```python
from build123d import *

# Parameters (mm, degrees)
F1_DEPTH = 50
F3_D     = 4.25


# Not quite as in the source:
# - a feature names something its author has since deleted; it is built from what else it names


with BuildPart() as f1:
    # F0 (on Top) → F1 (new body)
    with BuildSketch(Plane.XY):
        Polygon((-30.2708722231, 4.5814236456), (-30.2708722231, 0), (-30.2708722231, -1.8863187066), (-26.5, -1.8863187066), (-26.5, 0), (0, 0), (0, -26.5), (-26.5, -26.5), (-26.5, -22.9706130922), (-30.2708722231, -22.9706130922), (-30.2708722231, -26.5), (-30.2708722231, -29.9115763544), (0, -29.9115763544), (4.2217531975, -29.9115763544), (4.2217531975, 0), (4.2217531975, 4.5814236456), align=None)
        Polygon((-30.2708722231, -1.8863187066), (-30.2708722231, 0), (-30.2708722231, 4.5814236456), (-42.7924469113, 4.5814236456), (-42.7924469113, -1.8863187066), align=None)
        Polygon((-42.7924469113, -29.9115763544), (-30.2708722231, -29.9115763544), (-30.2708722231, -26.5), (-30.2708722231, -22.9706130922), (-42.7924469113, -22.9706130922), align=None)
        Polygon((0, -75.0411301851), (0, -29.9115763544), (-30.2708722231, -29.9115763544), align=None)
        Polygon((104.0906682611, -70.3669339418), (26.0842684656, -70.3669339418), (4.2217531975, -70.3669339418), (4.2217531975, -29.9115763544), (0, -29.9115763544), (0, -75.0411301851), (0, -85.0630626082), (104.0906682611, -78.3288473744), (104.0906682611, -75.0411301851), align=None)
        Polygon((26.0842684656, -70.3669339418), (4.2217531975, 4.5814236456), (4.2217531975, 0), (4.2217531975, -29.9115763544), (4.2217531975, -70.3669339418), align=None)
    extrude(amount=F1_DEPTH)

    # F3 (through all)
    with Locations(Plane(origin=(0, 4.5814236456, 0), x_dir=(-1, 0, 0), z_dir=(0, 1, 0))):
        with Locations((37.5032611191, 37.5), (37.5032611191, 12.5)):
            Hole(F3_D / 2)


solid = f1.part
```
For this review, take the finished solid that the model builds, in its own axes (mm). A direction names the side the tool comes from. Round coordinates to 2 decimals unless told otherwise and drop trailing zeros. Write each loop counter-clockwise with the first axis right and the second up, starting at its lowest first coordinate (ties: lowest second). Pieces come first, ordered by that corner, then holes.
1) Mouldability with a two-part tool opening along Z and no side actions: class faces 1 (the face through (-35, -22.971, 25)), 2 (the face through (-37.78, -26.49, 14.607)), 3 (the face through (9, -50, 0)) as +Z half, -Z half, draft (parallel to the pull), parting line (faces both ways), or undercut.
Answer below:
face 1: draft
face 2: undercut
face 3: -Z half
2) Take a section at A-A on z = 37.5. Give the boundary of the cut face in (x, y), then the cut area to 3 significant figures.
Answer below:
outline: (-42.79, -29.91) - (-39.63, -29.91) - (-39.63, -22.97) - (-42.79, -22.97) - close; (-42.79, -1.89) - (-39.63, -1.89) - (-39.63, 4.58) - (-42.79, 4.58) - close; (-35.38, -29.91) - (-30.27, -29.91) - (0, -75.04) - (0, -85.06) - (104.09, -78.33) - (104.09, -70.37) - (26.08, -70.37) - (4.22, 4.58) - (-35.38, 4.58) - (-35.38, -1.89) - (-26.5, -1.89) - (-26.5, 0) - (0, 0) - (0, -26.5) - (-26.5, -26.5) - (-26.5, -22.97) - (-35.38, -22.97) - close
area: 3,370 mm2
3) Machinability: for faces 4 (the face through (9, -50, 50)), 5 (the face through (0, -80, 25)), 6 (the face through (-26.5, -25, 25)), 7 (the face through (66, -70.367, 25)), which of the approach directions +Z, -Z, +X, -X, +Y, -Y give a long, thin tool a straight path to every point of the face, cutting with its end or side? Answer none if there is none.
Answer below:
face 4: +Z, +X, -X, +Y, -Y
face 5: +Z, -Z, -X, -Y
face 6: +Z, -Z
face 7: +Z, -Z, +X, +Y
4) Take a section at D-D on x = 16.5. Give the boundary of the cut face in (y, z), then the cut area to 3 significant figures.
Answer below:
outline: (-84, 0) - (-37.51, 0) - (-37.51, 50) - (-84, 50) - close
area: 2,320 mm2
5) For line 1 along Y through (x, z) = (-3, 19); line 2 along X through (y, z) = (2, 12); line 3 along X through (y, z) = (-14, 4), list the stretches that pass through material, from the lowest coordinate up.
Answer below:
line 1: y = -70.57 to -26.5, 0 to 4.58
line 2: x = -42.79 to -39.57, -35.44 to 4.97
line 3: x = 0 to 9.64
6) Take a section at C-C on y = -80. Give the boundary of the cut face in (x, z), then the cut area to 3 significant figures.
Answer below:
outline: (0, 0) - (78.26, 0) - (78.26, 50) - (0, 50) - close
area: 3,910 mm2
7) Take a section at B-B on z = 23. Give the boundary of the cut face in (x, y), then the cut area to 3 significant figures.
Answer below:
outline: (-42.79, -29.91) - (-30.27, -29.91) - (0, -75.04) - (0, -85.06) - (104.09, -78.33) - (104.09, -70.37) - (26.08, -70.37) - (4.22, 4.58) - (-42.79, 4.58) - (-42.79, -1.89) - (-26.5, -1.89) - (-26.5, 0) - (0, 0) - (0, -26.5) - (-26.5, -26.5) - (-26.5, -22.97) - (-42.79, -22.97) - close
area: 3,430 mm2
8) Insertion check: pin 1 Ø3 at (x, z) = (-27.5, 21.5) entering from -Y; pin 2 Ø5 at (y, z) = (-80.5, 24) entering from -X; pin 3 Ø15 at (x, z) = (69, 30.5) entering from +Y. Each pin has a flat end and moves straight along its axis. Give the tip position at first contact, or say it passes through.
Answer below:
pin 1: stops at y = -36.28
pin 2: stops at x = 0
pin 3: stops at y = -70.37
